Design review of the part shown in the three views and the two pictorial views. Dimensions are in mm from the part's minimum x, y and z. Round coordinates to 2 decimals unless told otherwise and drop trailing zeros. Loops run counter-clockwise (first coordinate to the right, second up) from the corner with the lowest first, then second, coordinate; pieces in that order, holes last. Notation, with made-up numbers: (43.5, 72) -> (47.5, 72) arc R22 cw to (47.5, 88) -> close; hole circle Ø4 at (61, 63). An arc over 180 degrees is marked (long way). Write each question's results on one line, items separated by ' | '. Start each with the question number.
Item 1: Clearance check with flat-ended pins moving along their axes: pin 1 Ø8 at (y, z) = (14.5, 12.5) entering from +X; pin 2 Ø6 at (y, z) = (24.5, 6.5) entering from -X; pin 3 Ø6 at (x, y) = (26, 5.5) entering from -Z; pin 4 Ø8 at (y, z) = (23.5, 13) entering from -X (1 decimal). State where each tip first meets the part, or that it passes through.
Item 2: We need section B-B (x = 28). Give the boundary of the cut face in (y, z).
Item 3: We need section A-A (z = 5). Give the boundary of the cut face in (x, y).
Item 4: We need section D-D (z = 7). Give the boundary of the cut face in (x, y).
Item 5: For L1, parallel to X at y = 17.5, z = 5.5; L2, parallel to Y at x = 17.5, z = 9.5, list the stretches that pass through material, from the lowest coordinate up. Write a range as from..to.
Item 6: Mouldability with a two-part tool opening along Y and no side actions: class the marked faces 1, 2 and 3 as pulls with the +Y half, pulls with the -Y half, needs draft (parallel to the pull), parting line crosses it, or undercut.
Item 7: We need section C-C (y = 11.5). Give the boundary of the cut face in (x, z).
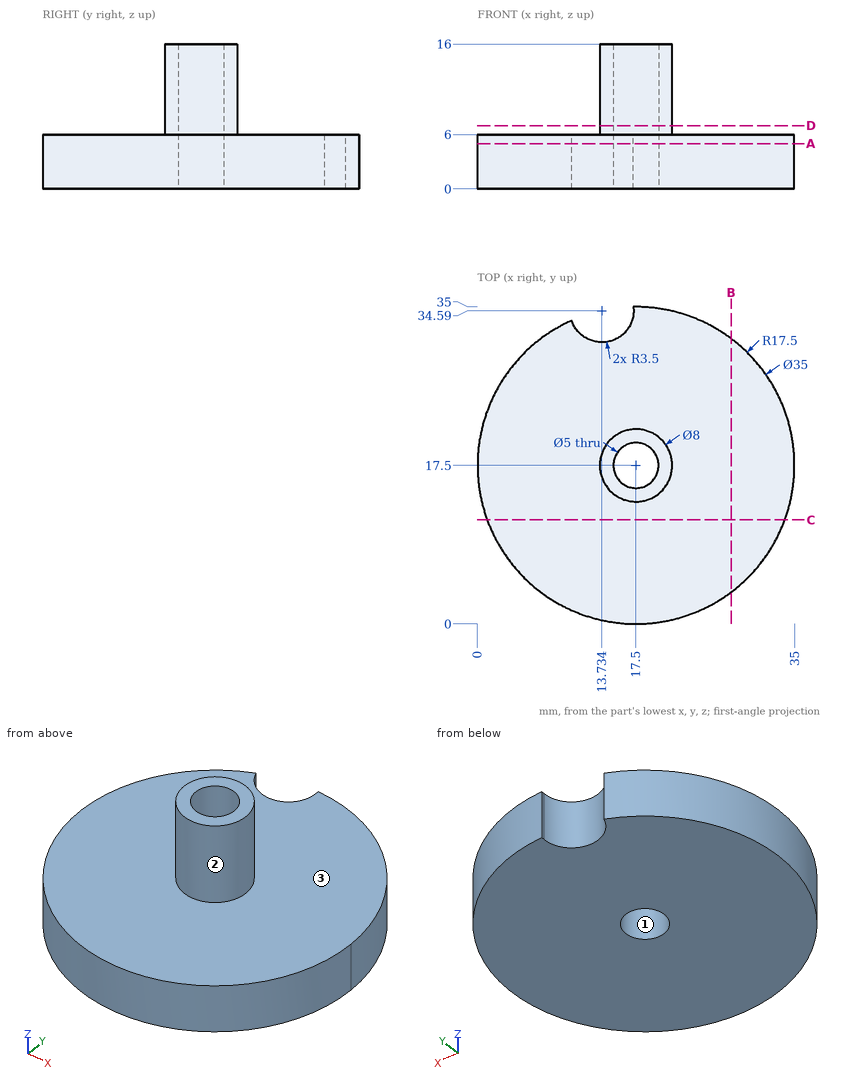
Here are the results:
1) pin 1: stops at x = 21.5 | pin 2: stops at x = 0.47 | pin 3: stops at z = 0 | pin 4: stops at x = 14
2) outline: (3.5, 0) -> (31.5, 0) -> (31.5, 6) -> (3.5, 6) -> close
3) outline: (10.41, 33.5) arc R17.5 ccw (long way) to (17.21, 35) arc R3.5 cw to (17.23, 34.59) arc R3.5 cw to start; hole circle Ø5 at (17.5, 17.5)
4) outline: circle Ø8 at (17.5, 17.5); hole circle Ø5 at (17.5, 17.5)
5) L1: x = 0..15, 20..35 | L2: y = 13.5..15, 20..21.5
6) face 1: undercut | face 2: parting line crosses it | face 3: needs draft
7) outline: (1.06, 0) -> (33.94, 0) -> (33.94, 6) -> (1.06, 6) -> close
